from build123d import *

# Parameters (mm, degrees)
SKETCH1_R           = 2
BOSS_EXTRUDE1_DEPTH = 1
SKETCH2_R           = 16
BOSS_EXTRUDE2_DEPTH = 13
SKETCH3_R           = 9.5
BOSS_EXTRUDE3_DEPTH = 2
FILLET1_R           = 5
FILLET2_R           = 2
SKETCH4_R           = 7.5
CUT_EXTRUDE1_DEPTH  = 11
FILLET3_R           = 7.5
FILLET4_R           = 1
FILLET5_R           = 1


with BuildPart() as part:
    # Sketch1 → Boss-Extrude1 (new body)
    with BuildSketch(Plane.XY):
        with BuildLine():
            Line((-12.6, 12.854571171), (-22.8, 2.856571371))
            ThreePointArc((-22.8, 2.856571371), (-24, 0), (-22.8, -2.856571371))
            Line((-22.8, -2.856571371), (-12.6, -12.854571171))
            ThreePointArc((-12.6, -12.854571171), (0, -18), (12.6, -12.854571171))
            Line((12.6, -12.854571171), (22.8, -2.856571371))
            ThreePointArc((22.8, -2.856571371), (24, 0), (22.8, 2.856571371))
            Line((22.8, 2.856571371), (12.6, 12.854571171))
            ThreePointArc((12.6, 12.854571171), (0, 18), (-12.6, 12.854571171))
        make_face()
        with Locations((-20, 0)):
            Circle(SKETCH1_R, mode=Mode.SUBTRACT)
        with Locations((20, 0)):
            Circle(SKETCH1_R, mode=Mode.SUBTRACT)
    extrude(amount=BOSS_EXTRUDE1_DEPTH)

    # Sketch2 → Boss-Extrude2 (add)
    with BuildSketch(Plane.XY.offset(1)):
        with Locations(Location((0, 0, 0), (0, 0, 180))):
            Circle(SKETCH2_R)
    extrude(amount=BOSS_EXTRUDE2_DEPTH)

    # Sketch3 → Boss-Extrude3 (add)
    with BuildSketch(Plane.XY.offset(14)):
        Circle(SKETCH3_R)
    extrude(amount=BOSS_EXTRUDE3_DEPTH)

    # Fillet1
    fillet1_edges = [part.edges().sort_by_distance(p)[0] for p in [
        (16, 0, 14),
    ]]
    fillet(fillet1_edges, radius=FILLET1_R)

    # Fillet2
    fillet2_edges = [part.edges().sort_by_distance(p)[0] for p in [
        (-9.5, 0, 14),
    ]]
    fillet(fillet2_edges, radius=FILLET2_R - 0.0001)  # a hair under: the kernel refuses the full size

    # Sketch4 → Cut-Extrude1 (cut)
    with BuildSketch(Plane.XY.offset(16)):
        Circle(SKETCH4_R)
    extrude(amount=-CUT_EXTRUDE1_DEPTH, mode=Mode.SUBTRACT)

    # Fillet3
    fillet3_edges = [part.edges().sort_by_distance(p)[0] for p in [
        (-7.5, 0, 5),
    ]]
    fillet(fillet3_edges, radius=FILLET3_R)

    # Fillet4
    fillet4_edges = [part.edges().sort_by_distance(p)[0] for p in [
        (-9.5, 0, 16),
    ]]
    fillet(fillet4_edges, radius=FILLET4_R)

    # Fillet5
    fillet5_edges = [part.edges().sort_by_distance(p)[0] for p in [
        (-7.5, 0, 16),
    ]]
    fillet(fillet5_edges, radius=FILLET5_R)


solid = part.part
Design review of the part built by this model. Coordinates are the model's own, in mm. A direction names the side the tool comes from. Coordinates: 2 decimals unless noted, no trailing zeros. Order: outer loops, then holes, each group sorted by start corner. A loop starts at its lowest first (then second) coordinate and runs counter-clockwise, first axis right, second up.
Item 1: For line 1 (Y direction, x = -20, z = 0.55); line 2 (Z direction, x = 10.5, y = -14.5); line 3 (Y direction, x = -4.5, z = 11), list the stretches that pass through material, from the lowest coordinate up.
Item 2: Take a section at C-C, the plane z = 3.25. Write out the cut boundary in (x, y).
Item 3: Take a section at B-B, the plane z = 8. Write out the cut boundary in (x, y).
Item 4: For pin 1 Ø5 at (y, z) = (-6, 2.5) entering from -X; pin 2 Ø6 at (x, z) = (13, 13.5) entering from +Y; pin 3 Ø3.5 at (x, y) = (-20, 0) entering from +Z; pin 4 Ø4.5 at (x, y) = (20, 0) entering from +Z, all flat-tipped, find the tip position at first contact; note any pin that passes through.
Item 5: Take a section at A-A, the plane x = 20. Write out the cut boundary in (y, z).
Item 6: The part is to be moulded in two halves that separate along X. For faces 1 (the cylindrical face through (18.4, -1.2, 0.5)), 2 (the flat face through (-17.771, -7.786, 0.493)), 3 (the flat face through (17.771, 7.786, 0.493)), say which applies: pulls with the +X half, pulls with the -X half, needs draft (parallel to the pull), parting line crosses it, or undercut.
Item 7: For faces 4 (the cylindrical face through (0.2, 18, 0.5)), 5 (the cylindrical face through (-7.493, 0.33, 13.768)), list the 3-axis set-ups (+Z, -Z, +X, -X, +Y, -Y) from which the entire face can be reached by the end or side of a thin tool; tool diameter is ignored.
The answers:
1. line 1: y = -5.6 to -2, 2 to 5.6
1. line 2: z = 0 to 1
1. line 3: y = -14.92 to -5.81, 5.81 to 14.92
2. outline: circle Ø32 at (0, 0)
3. outline: circle Ø32 at (0, 0); hole circle Ø12 at (0, 0)
4. pin 1: stops at x = -21.63
4. pin 2: stops at y = 10.92
4. pin 3: passes through
4. pin 4: stops at z = 1
5. outline: (-5.6, 0) - (-2, 0) - (-2, 1) - (-5.6, 1) - close; (2, 0) - (5.6, 0) - (5.6, 1) - (2, 1) - close
6. face 1: undercut
6. face 2: pulls with the -X half
6. face 3: pulls with the +X half
7. face 4: +Z, -Z, +Y
7. face 5: +Z
